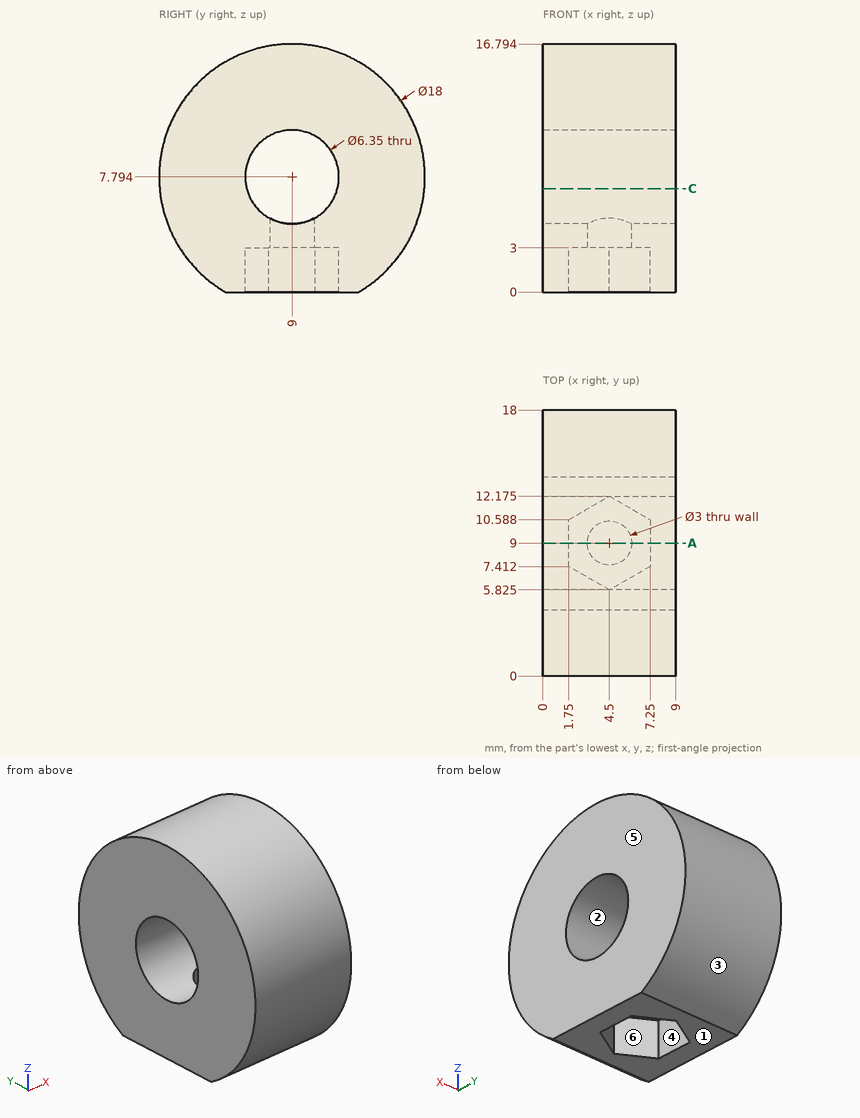
For this review, use the dimensioned drawing (mm, ordinates from the lowest corner) and the shaded views. A direction names the side the tool comes from. Give positions to 0.01 mm unless a question says otherwise; leave off trailing zeros. Order: outer loops, then holes, each group sorted by start corner. A loop starts at its lowest first (then second) coordinate and runs counter-clockwise, first axis right, second up. Notation, with made-up numbers: (8.25, 40) - (48.25, 40) arc R18 cw to (48.25, 73) - close; hole circle Ø9 at (26.5, -13.75). An arc over 180 degrees is marked (long way). Use CSV: the item, a comma, the result in double quotes. Start each with the question number.
Q1. Machinability: for the marked faces 5 and 6, which of the approach directions +Z, -Z, +X, -X, +Y, -Y give a long, thin tool a straight path to every point of the face, cutting with its end or side? Answer none if there is none.
Q2. For P1, Ø3, axis at x = 6, y = 10, coming from the -Z side; P2, Ø5, axis at x = 7, z = 14, coming from the +Y side; P3, Ø1, axis at x = 6.5, y = 8.5, coming from the -Z side; P4, Ø1, axis at x = 2, y = 6.5, coming from the +Z side, all flat-tipped, find the tip position at first contact; note any pin that passes through.
Q3. For line 1 (X direction, y = 7.5, z = 1.75); line 2 (Z direction, x = 8, y = 8.5); line 3 (Y direction, x = 1.5, z = 5) (1 decimal), list the stretches that pass through material, from the lowest coordinate up.
Q4. Take a section at C-C (z = 7). State the section outline as (x, y) points (1 decimal), and give its area (3 significant figures).
Q5. Take a section at A-A (y = 9). Count the separate pieces of the cut face and the enclosed holes in it.
Q6. Draft analysis for pull direction Z (two halves, no side actions). For the marked faces 1, 2, 3 and 4, state which applies: pulls with the +Z half, pulls with the -Z half, needs draft (parallel to the pull), parting line crosses it, or undercut.
Calculated:
1,face 5,"+Z, -Z, +X, +Y, -Y"
1,face 6,"-Z"
2,P1,"stops at z = 0"
2,P2,"stops at y = 17.2"
2,P3,"stops at z = 3"
2,P4,"stops at z = 16.57"
3,line 1,"x = 0 to 1.75, 7.25 to 9"
3,line 2,"z = 0 to 4.66, 10.93 to 16.78"
3,line 3,"y = 0.4 to 7.5, 10.5 to 17.6"
4,outline,"(0, 0) - (9, 0) - (9, 5.9) - (0, 5.9) - close; (0, 12.1) - (9, 12.1) - (9, 18) - (0, 18) - close"
4,area,"106 mm²"
5,separate pieces,"3"
5,enclosed holes,"0"
6,face 1,"pulls with the -Z half"
6,face 2,"undercut"
6,face 3,"parting line crosses it"
6,face 4,"needs draft"
